Job drawing, mm, ordinate dimensions from the low corner. One solid piece. A direction names the side the tool comes from. Round coordinates to 2 decimals unless told otherwise and drop trailing zeros. Loops run counter-clockwise (first coordinate to the right, second up) from the corner with the lowest first, then second, coordinate; pieces in that order, holes last. Notation, with made-up numbers: M -30.5,18.25 L 17.5,18.25 A14 cw 17.5,33.25 Z; hole C -11,-38 d8. An arc over 180 degrees is marked long. Use one line per item in the form item = value.
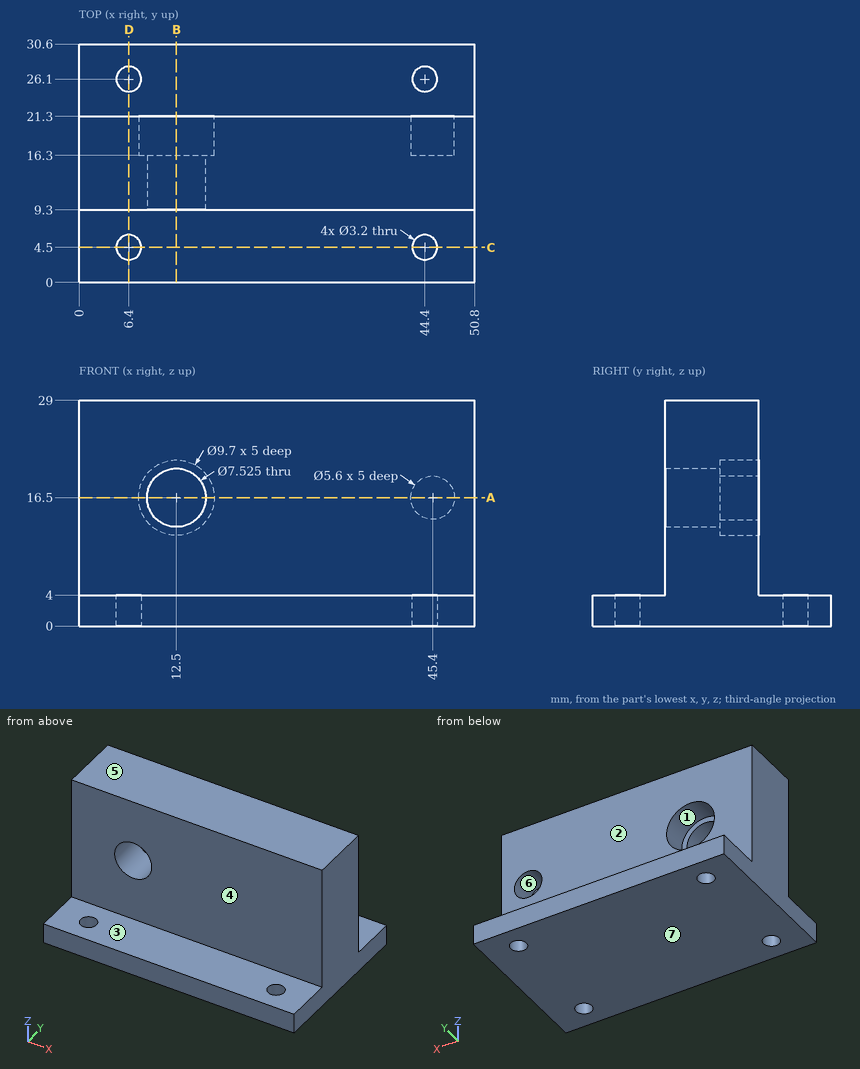
1. Tool access for the marked faces 1, 2 and 3: list every direction of +Z, -Z, +X, -X, +Y, -Y with a clear straight run to the whole face (end or side of a thin tool).
Completed:
face_1 = +Y
face_2 = +Z, +X, -X, +Y
face_3 = +Z, +X, -X, -Y
2. Drop flat-ended pins along their axis: P1, Ø12.5, axis at x = 22.5, z = 19, coming from the +Y side; P2, Ø3, axis at x = 28.5, y = 26, coming from the +Z side; P3, Ø8, axis at x = 13, z = 16.5, coming from the +Y side. Give the stop position or say it passes through.
Completed:
P1 = 21.3
P2 = 4
P3 = 16.3
3. Cut at C-C on y = 4.5. Write the cut outline in (x, z), and give its area (3 significant figures).
Completed:
outline = M 0,0 L 4.8,0 L 4.8,4 L 0,4 Z; M 8,0 L 42.8,0 L 42.8,4 L 8,4 Z; M 46,0 L 50.8,0 L 50.8,4 L 46,4 Z
area = 178 mm2
4. Cut at A-A on z = 16.5. Write the cut outline in (x, y), and give its area (3 significant figures).
Completed:
outline = M 0,9.3 L 8.74,9.3 L 8.74,16.3 L 7.65,16.3 L 7.65,21.3 L 0,21.3 Z; M 16.26,9.3 L 50.8,9.3 L 50.8,21.3 L 48.2,21.3 L 48.2,16.3 L 42.6,16.3 L 42.6,21.3 L 17.35,21.3 L 17.35,16.3 L 16.26,16.3 Z
area = 480 mm2
5. Pull direction Z, two halves, no side cores. Call the marked faces 4, 5, 6 and 7: +Z half, -Z half, draft (parallel to the pull), parting line (faces both ways), or undercut.
Completed:
face_4 = draft
face_5 = +Z half
face_6 = undercut
face_7 = -Z half
6. Cut at B-B on x = 12.5. Write the cut outline in (y, z).
Completed:
outline = M 0,0 L 30.6,0 L 30.6,4 L 21.3,4 L 21.3,11.65 L 16.3,11.65 L 16.3,12.74 L 9.3,12.74 L 9.3,4 L 0,4 Z; M 9.3,20.26 L 16.3,20.26 L 16.3,21.35 L 21.3,21.35 L 21.3,29 L 9.3,29 Z
7. Probe line 1 along Y through (x, z) = (6.4, 2.7); line 2 along Z through (x, y) = (47, 25); line 3 along Y through (x, z) = (10, 12). List the from-to ranges inside material, lowest first. Write a range as from..to.
Completed:
line_1 = 0..2.9, 6.1..24.5, 27.7..30.6
line_2 = 0..4
line_3 = 9.3..21.3
8. Cut at D-D on x = 6.4. Write the cut outline in (y, z), and give its area (3 significant figures).
Completed:
outline = M 0,0 L 2.9,0 L 2.9,4 L 0,4 Z; M 6.1,0 L 24.5,0 L 24.5,4 L 21.3,4 L 21.3,29 L 9.3,29 L 9.3,4 L 6.1,4 Z; M 27.7,0 L 30.6,0 L 30.6,4 L 27.7,4 Z
area = 397 mm2
